Here's the drawing with two shaded views (mm, measured from the low corner). I have some questions. Give positions to 0.01 mm unless a question says otherwise; leave off trailing zeros. Write each loop counter-clockwise with the first axis right and the second up, starting at its lowest first coordinate (ties: lowest second). Pieces come first, ordered by that corner, then holes.
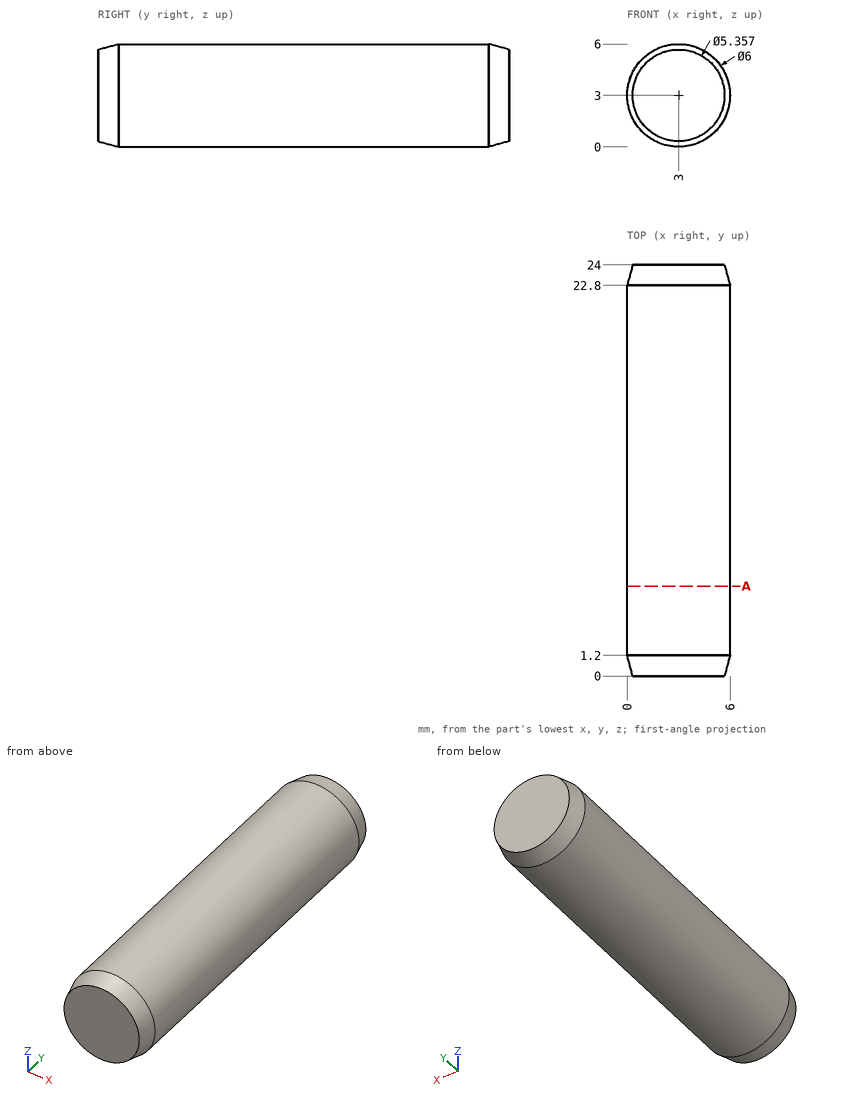
(1) Imagine slicing it at A-A, the plane y = 5.25. Write out the boundary of the cut face in (x, z), plus the area to 3 significant figures.
Returned:
outline: circle Ø6 at (3, 3)
area: 28.3 mm2
(2) If I drill on L1, parallel to Z at x = 1.45, y = 15.25; L2, parallel to Z at x = 1.2, y = 14.25; L3, parallel to X at y = 3.5, z = 2.75, over which ranges is the centre line in solid material (lowest first)?
Returned:
L1: z = 0.43 to 5.57
L2: z = 0.6 to 5.4
L3: x = 0.01 to 5.99
(3) Will these pins go through, and if not, where does the flat tip stop? P1, Ø1.5, axis at y = 12, z = 1.5, coming from the +X side; P2, Ø1, axis at y = 3.5, z = 1.5, coming from the +X side.
Returned:
P1: stops at x = 5.9
P2: stops at x = 5.83
